Work out the finished part from the listing and answer in its coordinate system (mm). Round coordinates to 2 decimals unless told otherwise and drop trailing zeros. Order: outer loops, then holes, each group sorted by start corner. A loop starts at its lowest first (then second) coordinate and runs counter-clockwise, first axis right, second up. Notation, with made-up numbers: (-32.75, 3) - (24.25, 3) arc R13 cw to (24.25, 14) - close; hole circle Ø2 at (-8, -15.5). An arc over 180 degrees is marked (long way). Put each result on its own line as item: value.
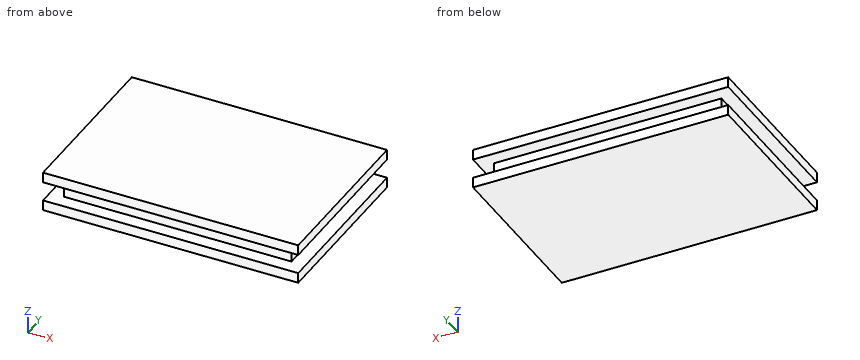
```python
from build123d import *

# Parameters (mm, degrees)
CROQUIS1_W              = 37
CROQUIS1_H              = 25
SALIENTE_EXTRUIR1_DEPTH = 1.5
CROQUIS2_W              = 33
CROQUIS2_H              = 21
SALIENTE_EXTRUIR2_DEPTH = 2.8
SALIENTE_EXTRUIR3_START = 4.3
CROQUIS1_2_W            = 37
CROQUIS1_2_H            = 25
SALIENTE_EXTRUIR3_DEPTH = 1.5


with BuildPart() as part:
    # Croquis1 → Saliente-Extruir1 (new body)
    with BuildSketch(Plane.XY):
        Rectangle(CROQUIS1_W, CROQUIS1_H)
    extrude(amount=SALIENTE_EXTRUIR1_DEPTH)

    # Croquis2 → Saliente-Extruir2 (add)
    with BuildSketch(Plane.XY.offset(1.5)):
        Rectangle(CROQUIS2_W, CROQUIS2_H)
    extrude(amount=SALIENTE_EXTRUIR2_DEPTH)

    # Croquis1<2> → Saliente-Extruir3 (add)
    with BuildSketch(Plane.XY.offset(SALIENTE_EXTRUIR3_START)):
        Rectangle(CROQUIS1_2_W, CROQUIS1_2_H)
    extrude(amount=SALIENTE_EXTRUIR3_DEPTH)


solid = part.part
```
1) Given pin 1 Ø2 at (y, z) = (3, 3) entering from +X, flat-ended and moving along its own axis, determine where the tip first touches the part or whether it passes through.
Findings below:
pin 1: stops at x = 16.5
2) A cutting plane is placed at C-C on z = 2.9. Write down the section's boundary in (x, y), then the cut area to 3 significant figures.
Findings below:
outline: (-16.5, -10.5) - (16.5, -10.5) - (16.5, 10.5) - (-16.5, 10.5) - close
area: 693 mm2
3) A cutting plane is placed at B-B on x = -16. Write down the section's boundary in (y, z).
Findings below:
outline: (-12.5, 0) - (12.5, 0) - (12.5, 1.5) - (10.5, 1.5) - (10.5, 4.3) - (12.5, 4.3) - (12.5, 5.8) - (-12.5, 5.8) - (-12.5, 4.3) - (-10.5, 4.3) - (-10.5, 1.5) - (-12.5, 1.5) - close
4) Straight lines are drawn through the part: L1, parallel to Z at x = 5, y = 11; L2, parallel to X at y = -4.5, z = 2.35; L3, parallel to Y at x = -10, z = 4.1. For each, find the intervals that lie inside material, in ascending order. Write a range as from..to.
Findings below:
L1: z = 0..1.5, 4.3..5.8
L2: x = -16.5..16.5
L3: y = -10.5..10.5
5) A cutting plane is placed at A-A on y = 8. Write down the section's boundary in (x, z).
Findings below:
outline: (-18.5, 0) - (18.5, 0) - (18.5, 1.5) - (16.5, 1.5) - (16.5, 4.3) - (18.5, 4.3) - (18.5, 5.8) - (-18.5, 5.8) - (-18.5, 4.3) - (-16.5, 4.3) - (-16.5, 1.5) - (-18.5, 1.5) - close
